Read the model definition and answer for the solid it produces. Units are mm, in the model's axes. Coordinates: 2 decimals unless noted, no trailing zeros. Order: outer loops, then holes, each group sorted by start corner. A loop starts at its lowest first (then second) coordinate and runs counter-clockwise, first axis right, second up. Notation, with made-up numbers: (17.5, 64.5) - (40.5, 64.5) arc R27 ccw to (40.5, 86.5) - close; hole circle Ø11 at (52, 74.5). An arc over 180 degrees is marked (long way). Use one line per item in the form item = value.
```python
from build123d import *

# Parameters (mm, degrees)
BOSS_EXTRUDE1_DEPTH  = 1
M3_CLEARANCE_HOLE1_D = 3.4


with BuildPart() as part:
    # Sketch1 → Boss-Extrude1 (new body)
    with BuildSketch(Plane.XY):
        Polygon((0, 0), (0, 100), (15, 100), (15, 15), (100, 15), (100, 0), align=None)
    extrude(amount=BOSS_EXTRUDE1_DEPTH)

    # M3 Clearance Hole1 (through all)
    with Locations(Plane(origin=(0, 0, 0), x_dir=(-1, 0, 0), z_dir=(0, 0, -1))):
        with Locations((-92.5, 7.5), (-7.5, 7.5), (-7.5, 92.5), (-7.5, 50), (-50, 7.5)):
            Hole(M3_CLEARANCE_HOLE1_D / 2)


solid = part.part
```
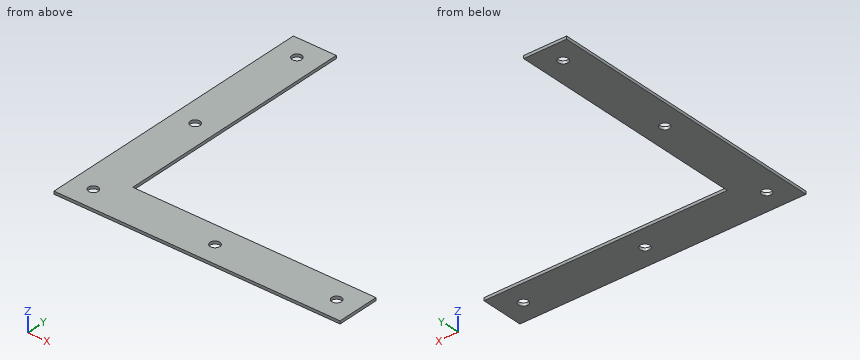
(1) Straight lines are drawn through the part: L1, parallel to Y at x = 7.5, z = 0.6; L2, parallel to X at y = 92.5, z = 0.7. For each, find the intervals that lie inside material, in ascending order.
Answer list:
L1 = 0 to 5.8, 9.2 to 48.3, 51.7 to 90.8, 94.2 to 100
L2 = 0 to 5.8, 9.2 to 15
(2) Section C-C, the plane z = 0.65 is taken. Write down the section's boundary in (x, y), then the cut area to 3 significant figures.
Answer list:
outline = (0, 0) - (100, 0) - (100, 15) - (15, 15) - (15, 100) - (0, 100) - close; hole circle Ø3.4 at (7.5, 7.5); hole circle Ø3.4 at (7.5, 50); hole circle Ø3.4 at (7.5, 92.5); hole circle Ø3.4 at (50, 7.5); hole circle Ø3.4 at (92.5, 7.5)
area = 2,730 mm2
(3) Section D-D, the plane x = 7.5 is taken. Write down the section's boundary in (y, z).
Answer list:
outline = (0, 0) - (5.8, 0) - (5.8, 1) - (0, 1) - close; (9.2, 0) - (48.3, 0) - (48.3, 1) - (9.2, 1) - close; (51.7, 0) - (90.8, 0) - (90.8, 1) - (51.7, 1) - close; (94.2, 0) - (100, 0) - (100, 1) - (94.2, 1) - close
(4) Section A-A, the plane x = 50 is taken. Write down the section's boundary in (y, z).
Answer list:
outline = (0, 0) - (5.8, 0) - (5.8, 1) - (0, 1) - close; (9.2, 0) - (15, 0) - (15, 1) - (9.2, 1) - close
(5) Given pin 1 Ø0.5 at (y, z) = (38, 0.5) entering from +X, flat-ended and moving along its own axis, determine where the tip first touches the part or whether it passes through.
Answer list:
pin_1 = 15
